Input: dimensioned drawing with shaded views. Units: mm. Origin: part minimum x, y, z. Round coordinates to 2 decimals unless told otherwise and drop trailing zeros. Loops run counter-clockwise (first coordinate to the right, second up) from the corner with the lowest first, then second, coordinate; pieces in that order, holes last. Notation, with made-up numbers: (1.25, 0.5) - (12.25, 0.5) arc R18 cw to (12.25, 33.5) - close; hole circle Ø4 at (29.5, -21). An arc over 180 degrees is marked (long way). One line per question, with ' | ' between items. Start each with the question number.
1. Cut plane D-D (z = 19.5). Return loops of the section in (x, y), then the cut area to 3 significant figures.
2. Pin query (flat end, axial travel): pin 1 (0.9 mm diameter, centred on y = 1, z = 101.5, fed in from +X); pin 2 (4 mm diameter, centred on x = 81, z = 53.5, fed in from -Y); pin 3 (0.9 mm diameter, centred on y = 2, z = 50, fed in from +X). Return the tip coordinate at first contact, or that it passes through.
3. Ray query, line 1 (X direction, y = 1.9, z = 49.5); line 2 (X direction, y = 1.9, z = 60); line 3 (X direction, y = 1.85, z = 114). Return the intervals inside material, ascending.
4. Cut plane B-B (x = 114). Return loops of the section in (y, z), then the cut area to 3 significant figures.
5. Cut plane C-C (y = 1.1). State how many separate pieces and enclosed holes the cut face has, then the cut area to 3 significant figures.
6. Cut plane A-A (z = 6). Return loops of the section in (x, y), then the cut area to 3 significant figures.
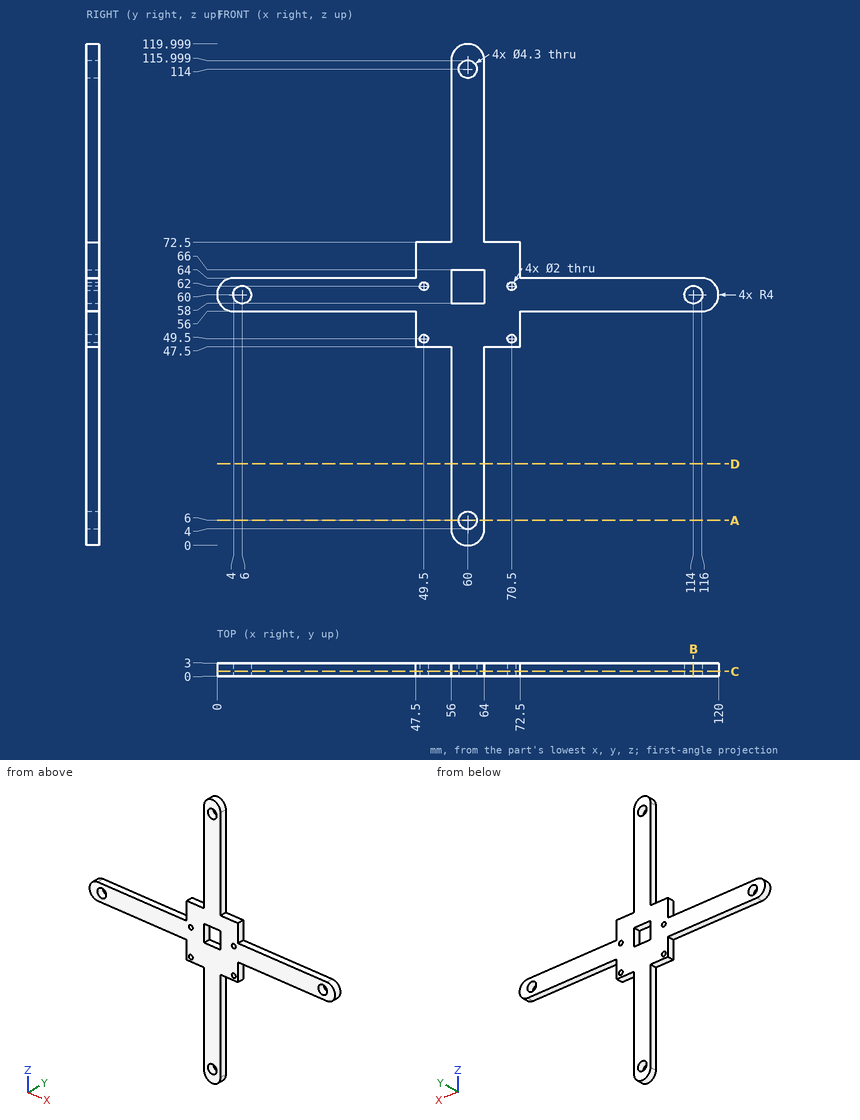
Answers follow:
1) outline: (56, 0) - (64, 0) - (64, 3) - (56, 3) - close | area: 24.0 mm2
2) pin 1: stops at x = 64 | pin 2: passes through | pin 3: stops at x = 72.5
3) line 1: x = 47.5 to 48.5, 50.5 to 69.5, 71.5 to 72.5 | line 2: x = 0 to 3.85, 8.15 to 56, 64 to 111.85, 116.15 to 120 | line 3: x = 56 to 57.85, 62.15 to 64
4) outline: (0, 56) - (3, 56) - (3, 57.85) - (0, 57.85) - close; (0, 62.15) - (3, 62.15) - (3, 64) - (0, 64) - close | area: 11.1 mm2
5) separate pieces: 1 | enclosed holes: 9 | area: 1,980 mm2
6) outline: (56, 0) - (57.85, 0) - (57.85, 3) - (56, 3) - close; (62.15, 0) - (64, 0) - (64, 3) - (62.15, 3) - close | area: 11.1 mm2
